Read the model definition and answer for the solid it produces. Units are mm, in the model's axes. A direction names the side the tool comes from. Coordinates: 2 decimals unless noted, no trailing zeros. Write each loop counter-clockwise with the first axis right and the second up, starting at its lowest first coordinate (ties: lowest second). Pieces come first, ordered by that corner, then holes. Notation, with made-up numbers: (29, -20.5) - (34, -20.5) arc R31 ccw to (34, 14.5) - close; hole circle Ø3 at (75.25, 58). An arc over 180 degrees is marked (long way). Return JSON: item names as keys, results as strings.
```python
from build123d import *

# Parameters (mm, degrees)
SKETCH_1_R          = 6
EXTRUDE_1_DEPTH     = 3
SKETCH_2_R          = 6
EXTRUDE_2_DEPTH     = 32
HOLE_WIZARD_M8_1_D  = 6.8
SKETCH_6_R          = 3
CUT_EXTRUDE_1_DEPTH = 10


with BuildPart() as part:
    # 草图1 → 凸台-拉伸1 (new body)
    with BuildSketch(Plane(origin=(0, 0, 0), x_dir=(1, 0, 0), z_dir=(0, 1, 0))):
        with Locations((-13.5, 0)):
            Circle(SKETCH_1_R)
        with BuildLine():
            Line((13.5, 6), (-13.5, 6))
            ThreePointArc((-13.5, 6), (-9.257359313, 4.242640687), (-7.5, 0))
            ThreePointArc((-7.5, 0), (-9.257359313, -4.242640687), (-13.5, -6))
            Line((-13.5, -6), (13.5, -6))
            ThreePointArc((13.5, -6), (7.5, 0), (13.5, 6))
        make_face()
        with Locations((13.5, 0)):
            Circle(SKETCH_1_R)
    extrude(amount=EXTRUDE_1_DEPTH)

    # 草图2 → 凸台-拉伸2 (add)
    with BuildSketch(Plane(origin=(0, 3, 0), x_dir=(1, 0, 0), z_dir=(0, 1, 0))):
        Circle(SKETCH_2_R)
    extrude(amount=EXTRUDE_2_DEPTH)

    # M8 螺纹孔1 (through all)
    with Locations(Plane(origin=(0, 35, 0), x_dir=(1, 0, 0), z_dir=(0, 1, 0))):
        with Locations((0, 0)):
            Hole(HOLE_WIZARD_M8_1_D / 2)

    # 草图6 → 切除-拉伸1 (cut)
    with BuildSketch(Plane(origin=(0, 3, 0), x_dir=(1, 0, 0), z_dir=(0, 1, 0))):
        with Locations((-13.5, 0)):
            Circle(SKETCH_6_R)
        with Locations((13.5, 0)):
            Circle(SKETCH_6_R)
    extrude(amount=-CUT_EXTRUDE_1_DEPTH, mode=Mode.SUBTRACT)


solid = part.part
```
(1) A cutting plane is placed at D-D (z = 5). Determine the outline of the cut face in (x, y).
Answer:
{"outline": "(-16.82, 0) - (16.82, 0) - (16.82, 3) - (3.32, 3) - (3.32, 35) - (-3.32, 35) - (-3.32, 3) - (-16.82, 3) - close"}
(2) A cutting plane is placed at A-A (z = 0). Determine the outline of the cut face in (x, y), and give its area (3 significant figures).
Answer:
{"outline": "(-19.5, 0) - (-16.5, 0) - (-16.5, 3) - (-19.5, 3) - close; (-10.5, 0) - (-3.4, 0) - (-3.4, 35) - (-6, 35) - (-6, 3) - (-10.5, 3) - close; (3.4, 0) - (10.5, 0) - (10.5, 3) - (6, 3) - (6, 35) - (3.4, 35) - close; (16.5, 0) - (19.5, 0) - (19.5, 3) - (16.5, 3) - close", "area": "227 mm²"}
(3) Flat-ended cylindrical pins translate along their axes: P1, Ø8, axis at x = -14.5, y = 9.5, coming from the +Z side; P2, Ø2, axis at y = 16, z = -0.5, coming from the +X side; P3, Ø2, axis at x = -3.5, y = 28, coming from the -Z side; P4, Ø4, axis at y = 25.5, z = -3.5, coming from the +X side. Find the tip coordinate at first contact, or state that the pin passes through.
Answer:
{"P1": "through", "P2": "x = 6", "P3": "z = -5.45", "P4": "x = 5.81"}
(4) Determine the mould class of faces 3 (the face through (-10, 3, 0)), 4 (the face through (-19.5, 1.5, -0.1)), 5 (the face through (0.74, 17.25, 3.32)) for opening direction X: +X half, -X half, draft (parallel to the pull), parting line (faces both ways), or undercut.
Answer:
{"face 3": "draft", "face 4": "-X half", "face 5": "undercut"}
(5) Straight lines are drawn through the part: line 1 (Z direction, x = 0, y = 16); line 2 (Z direction, x = 13.5, y = 1.6); line 3 (X direction, y = 2.5, z = 0.75). For each, find the intervals that lie inside material, in ascending order. Write a range as from..to.
Answer:
{"line 1": "-6..-3.4, 3.4..6", "line 2": "-6..-3, 3..6", "line 3": "-19.45..-16.4, -10.6..-3.32, 3.32..10.6, 16.4..19.45"}
(6) Which of the six approach directions +Z, -Z, +X, -X, +Y, -Y give full straight-line access (tool end or side, diameter ignored) to faces 1 (the face through (-6, 19, 0)), 2 (the face through (10.5, 1.5, -0.1))?
Answer:
{"face 1": "+Y", "face 2": "+Y, -Y"}
(7) A cutting plane is placed at C-C (y = 13). Determine the outline of the cut face in (x, z).
Answer:
{"outline": "circle Ø12 at (0, 0); hole circle Ø6.8 at (0, 0)"}
(8) A cutting plane is placed at B-B (x = 12.5). Determine the outline of the cut face in (y, z).
Answer:
{"outline": "(0, -6) - (3, -6) - (3, -2.83) - (0, -2.83) - close; (0, 2.83) - (3, 2.83) - (3, 6) - (0, 6) - close"}
